from build123d import *

# Parameters (mm, degrees)
SKETCH1_R           = 14.224
EXTRUDE1_DEPTH      = 71.4375
EXTRUDE1_DEPTH_BACK = 71.4375
SKETCH3_W           = 0.762
SKETCH3_H           = 0.762
RODHOLE_START       = -112.0375
SKETCH8_R           = 3.9624
RODHOLE_DEPTH       = 112.0375
SKETCH9_R           = 13.49375
STROKECHAMBER_DEPTH = 55.8
CHAMFER1_SIZE       = 0.5
SKETCH4_W           = 3.048
SKETCH4_H           = 12.7
SKETCH4_W_2         = 0.5
SKETCH4_H_2         = 6.096
FLATS_DEPTH         = 15.2240001
FLATS_DEPTH_BACK    = 15.2240001
SKETCH12_W          = 9.398
SKETCH12_H          = 15.375
ENDFLATS_DEPTH      = 15.2240001
ENDFLATS_DEPTH_BACK = 15.2240001


with BuildPart() as part:
    # Sketch1 → Extrude1 (new body, two sides)
    with BuildSketch(Plane.XY) as extrude1_sk:
        Circle(SKETCH1_R)
    extrude(amount=EXTRUDE1_DEPTH)
    extrude(extrude1_sk.sketch, amount=-EXTRUDE1_DEPTH_BACK)

    # Sketch2 → Nose (revolve)
    with BuildSketch(Plane(origin=(0, 0, 0), x_dir=(0, 0, -1), z_dir=(1, 0, 0))):
        Polygon((-71.4375, 7.9248), (-73.7235, 7.9248), (-73.7235, 7), (-76.5235, 7), (-76.5235, 7.9375), (-84.1375, 7.9375), (-84.1375, 0), (-71.4375, 0), align=None)
    revolve(axis=Axis((0, 0, 0), (0, 0, 1)))

    # Sketch3 → CoverGrooves (revolve, cut)
    with BuildSketch(Plane(origin=(0, 0, 0), x_dir=(0, 0, -1), z_dir=(1, 0, 0))):
        with Locations((-50.038, 13.843)):
            Rectangle(SKETCH3_W, SKETCH3_H)
        Polygon((-48.895, 14.224), (-48.895, 13.462), (-48.133, 13.462), (-47.371, 14.224), align=None)
        Polygon((37.7405, 14.224), (37.7405, 13.462), (36.9785, 14.224), align=None)
        Polygon((36.2165, 14.224), (36.2165, 13.462), (35.4545, 14.224), align=None)
    revolve(axis=Axis((0, 0, 0), (0, 0, 1)), mode=Mode.SUBTRACT)

    # Sketch7 → FrontPort (revolve, cut)
    with BuildSketch(Plane(origin=(0, 0, 0), x_dir=(0, 0, -1), z_dir=(1, 0, 0))):
        Polygon((-57.4675, 14.224), (-51.6175, 14.224), (-52.3175, 13.524), (-52.3175, 0), (-57.4675, 0), align=None)
    revolve(axis=Axis((0, 0, 57.4675), (0, 1, 0)), mode=Mode.SUBTRACT)

    # Sketch8 → RodHole (cut)
    with BuildSketch(Plane.XY.offset(84.1375).offset(RODHOLE_START)):
        Circle(SKETCH8_R)
    extrude(amount=RODHOLE_DEPTH, mode=Mode.SUBTRACT)

    # Sketch9 → StrokeChamber (cut)
    with BuildSketch(Plane.XY.offset(-27.9)):
        Circle(SKETCH9_R)
    extrude(amount=STROKECHAMBER_DEPTH, mode=Mode.SUBTRACT)

    # Chamfer1
    chamfer1_edges = [part.edges().sort_by_distance(p)[0] for p in [
        (-14.224, 0, -71.4375),
        (-3.9624, 0, 84.1375),
        (-14.224, 0, 71.4375),
        (0, -7.9375, 84.1375),
    ]]
    chamfer(chamfer1_edges, length=CHAMFER1_SIZE)

    # Sketch4 → Flats (cut, two sides)
    with BuildSketch(Plane(origin=(0, 0, 0), x_dir=(1, 0, 0), z_dir=(0, 1, 0))) as flats_sk:
        with Locations((12.7, -65.0875)):
            Rectangle(SKETCH4_W, SKETCH4_H)
        with Locations((13.974, 68.3895)):
            Rectangle(SKETCH4_W_2, SKETCH4_H_2)
        with Locations((-13.974, 68.3895)):
            Rectangle(SKETCH4_W_2, SKETCH4_H_2)
        with Locations((-12.7, -65.0875)):
            Rectangle(SKETCH4_W, SKETCH4_H)
    extrude(amount=FLATS_DEPTH, mode=Mode.SUBTRACT)
    extrude(flats_sk.sketch, amount=-FLATS_DEPTH_BACK, mode=Mode.SUBTRACT)

    # Sketch11 → EndThreads (revolve, cut)
    with BuildSketch(Plane(origin=(0, 0, 0), x_dir=(0, 0, -1), z_dir=(1, 0, 0))):
        Polygon((71.4375, 7.4375), (70.9375, 7.9375), (58.9431, 7.9375), (58.9431, 7), (57.9755, 7), (57.9755, 7.9375), (55.6895, 7.9375), (55.6895, 13.462), (54.9275, 14.224), (71.4375, 14.224), align=None)
    revolve(axis=Axis((0, 0, 0), (0, 0, -1)), mode=Mode.SUBTRACT)

    # Sketch13 → RearTopPort (revolve, cut)
    with BuildSketch(Plane(origin=(0, 0, 0), x_dir=(0, 0, -1), z_dir=(1, 0, 0))):
        Polygon((48.5794, 0), (53.7294, 0), (53.7294, 13.524), (54.4294, 14.224), (48.5794, 14.224), align=None)
    revolve(axis=Axis((0, 0, -48.5794), (0, 1, 0)), mode=Mode.SUBTRACT)

    # Sketch12 → EndFlats (cut, two sides)
    with BuildSketch(Plane(origin=(0, 0, 0), x_dir=(0, -1, 0), z_dir=(1, 0, 0))) as endflats_sk:
        with Locations((9.525, 63.75)):
            Rectangle(SKETCH12_W, SKETCH12_H)
        with Locations((-9.525, 63.75)):
            Rectangle(SKETCH12_W, SKETCH12_H)
    extrude(amount=ENDFLATS_DEPTH, mode=Mode.SUBTRACT)
    extrude(endflats_sk.sketch, amount=-ENDFLATS_DEPTH_BACK, mode=Mode.SUBTRACT)

    # Sketch15 → ClevisPinHole (revolve, cut)
    with BuildSketch(Plane(origin=(0, 0, 0), x_dir=(0, -1, 0), z_dir=(1, 0, 0))):
        Polygon((4.826, 68.0132), (4.326, 67.5132), (-4.326, 67.5132), (-4.826, 68.0132), (-4.826, 64.3255), (4.826, 64.3255), align=None)
    revolve(axis=Axis((0, 0, -64.3255), (0, -1, 0)), mode=Mode.SUBTRACT)

    # Sketch18 → ClevisPin (revolve)
    with BuildSketch(Plane(origin=(0, 0, 0), x_dir=(0, 0, -1), z_dir=(1, 0, 0))):
        Polygon((64.3255, 9.525), (67.0132, 9.525), (67.5132, 9.025), (67.5132, -9.025), (67.0132, -9.525), (64.3255, -9.525), align=None)
    revolve(axis=Axis((0, 0, -64.3255), (0, 1, 0)))


solid = part.part
Verification items for the finished model (mm, model axes). A direction names the side the tool comes from. Coordinates: 2 decimals unless noted, no trailing zeros. Order: outer loops, then holes, each group sorted by start corner. A loop starts at its lowest first (then second) coordinate and runs counter-clockwise, first axis right, second up. Notation, with made-up numbers: M -14,-2 L 33,-2 A18 cw 33,15 Z; hole C -35,42 d8. An arc over 180 degrees is marked long. Write each question's results on one line, items separated by ' | '.
1) Access from +Z, -Z, +X, -X, +Y, -Y to the whole of each face (thin tool, end or side, straight path). Record for faces 4 (the face through (7.75, -1.72, 80.13)), 5 (the face through (11.176, 0, 65)), 6 (the face through (0, -9.525, -64)).
Solved:
face 4: +Z | face 5: +Z, +X, +Y, -Y | face 6: -Z, +X, -X, -Y
2) Section check A-A on z = 14. Record the cut outline in (x, y), plus the area to 3 significant figures.
Solved:
outline: C 0,0 d28.45; hole C 0,0 d26.99 | area: 63.6 mm²
3) Release check for a two-part mould opening along Y. For faces 1 (the face through (0, 0, -27.9)), 2 (the face through (13, -5, 50.419)), 3 (the face through (8.191, -10.683, 50.033)) record: pulls with the +Y half, pulls with the -Y half, needs draft (parallel to the pull), parting line crosses it, or undercut.
Solved:
face 1: undercut | face 2: needs draft | face 3: parting line crosses it
4) Scan lines: line 1 along Z through (x, y) = (-6.75, -3); line 2 along Z through (x, y) = (11.75, -1); line 3 along Z through (x, y) = (3.5, 7.25). Record each from-to range of solid material in increasing order. Write a range as [from, to].
Solved:
line 1: z = [-71.44, -58.94], [-57.98, -27.9], [27.9, 73.72], [76.52, 84.14] | line 2: z = [-55.69, -27.9], [27.9, 58.74] | line 3: z = [-55.69, -52.36], [-44.8, -27.9], [27.9, 53.69], [61.25, 71.44]
5) Gauge pin test, flat ends, axial feed: pin 1 Ø1 at (y, z) = (10.5, 46) entering from -X; pin 2 Ø4 at (y, z) = (9.5, -4) entering from -X; pin 3 Ø0.9 at (x, y) = (12.5, 4) entering from +Z. Record the tip position at first contact, or that the pin passes through.
Solved:
pin 1: stops at x = -10.12 | pin 2: stops at x = -12.09 | pin 3: stops at z = 58.74
6) Section check B-B on y = 12. Give the number of separate pieces and of enclosed holes in the cut face, plus the area to 3 significant figures.
Solved:
separate pieces: 1 | enclosed holes: 3 | area: 1,080 mm²
7) Section check C-C on z = -49. Record the cut outline in (x, y).
Solved:
outline: M -5.13,0 L -5.13,13.27 A14.22 ccw long 5.13,13.27 L 5.13,0 Z
